```python
from build123d import *

# Parameters (mm, degrees)
F1_DEPTH       = 15
F1_DEPTH_BACK  = 5
F2_START       = 11
F2_DEPTH       = 4
F3_DEPTH       = 5
F4_D           = 3.8
F4_CSINK_D     = 8.5
F4_CSINK_ANGLE = 90
F5_SIZE        = 1.5


with BuildPart() as f1:
    # F0 (on Top) → F1 (new body, two sides)
    with BuildSketch(Plane.XY) as f1_sk:
        with BuildLine():
            ThreePointArc((7.3, 0), (0, -7.3), (-7.3, 0))
            Line((-7.3, 0), (-7.3, 8))
            Line((-7.3, 8), (-10.3, 8))
            Line((-10.3, 8), (-10.3, 0))
            ThreePointArc((-10.3, 0), (0, -10.3), (10.3, 0))
            Line((10.3, 0), (10.3, 8))
            Line((10.3, 8), (7.3, 8))
            Line((7.3, 8), (7.3, 0))
        make_face()
    extrude(amount=F1_DEPTH)
    extrude(f1_sk.sketch, amount=-F1_DEPTH_BACK)

    # F0 (on Top) → F2 (join)
    with BuildSketch(Plane.XY.offset(F2_START)):
        Polygon((-7.3, 8), (-7.3, 0), (-7, 0.7787641953), (-7, 8), align=None)
        Polygon((7, 0.7787641953), (7.3, 0), (7.3, 8), (7, 8), align=None)
    extrude(amount=F2_DEPTH)

    # F0 (on Top) → F3 (join)
    with BuildSketch(Plane.XY):
        Polygon((-7.3, 8), (-7.3, 0), (-7, 0.7787641953), (-7, 8), align=None)
        with BuildLine():
            Line((-7, 0.7787641953), (-7.3, 0))
            ThreePointArc((-7.3, 0), (0, -7.3), (7.3, 0))
            Line((7.3, 0), (7, 0.7787641953))
            Line((7, 0.7787641953), (7, 8))
            Line((7, 8), (7.3, 8))
            Line((7.3, 8), (10.3, 8))
            Line((10.3, 8), (10.3, 16))
            ThreePointArc((10.3, 16), (0, 26.3), (-10.3, 16))
            Line((-10.3, 16), (-10.3, 8))
            Line((-10.3, 8), (-7.3, 8))
            Line((-7.3, 8), (-7, 8))
            Line((-7, 8), (-7, 0.7787641953))
        make_face()
        Polygon((7, 0.7787641953), (7.3, 0), (7.3, 8), (7, 8), align=None)
    extrude(amount=-F3_DEPTH)

    # F4 (through all)
    with Locations(Plane.XY):
        with Locations((0, 16), (0, 0)):
            CounterSinkHole(F4_D / 2, F4_CSINK_D / 2, counter_sink_angle=F4_CSINK_ANGLE)

    # F5
    f5_edges = [f1.edges().sort_by_distance(p)[0] for p in [
        (-7, 8, 13),
        (7, 8, 13),
    ]]
    chamfer(f5_edges, length=F5_SIZE)


solid = f1.part
```
Check sheet for the modelled part. Datum: model origin and axes. Units: mm. A direction names the side the tool comes from. Coordinates: 2 decimals unless noted, no trailing zeros. Order: outer loops, then holes, each group sorted by start corner. A loop starts at its lowest first (then second) coordinate and runs counter-clockwise, first axis right, second up. Notation, with made-up numbers: (-36, 71.5) -> (-24, 71.5) arc R28 cw to (-24, 105.5) -> close; hole circle Ø10 at (-5, 14). An arc over 180 degrees is marked (long way). Write item = value, one per line. Start each with the question number.
1) Access from +Z, -Z, +X, -X, +Y, -Y to the whole of each face (thin tool, end or side, straight path). Record for faces 1 (the flat face through (0, 8, -5)), 2 (the cylindrical face through (1.9, 0.08, -3.69)), 3 (the flat face through (7.3, 3, 6)), 4 (the flat face through (-9, 8, 7)), 5 (the flat face through (-7.9, 7.4, 7.4)).
2) Go/stop test with flat-tipped pins: P1, Ø1, axis at x = 6.5, z = 5.5, coming from the -Y side; P2, Ø12, axis at y = 15.5, z = 11.5, coming from the -X side; P3, Ø4.5, axis at x = 0, y = 16, coming from the +Z side; P4, Ø0.9, axis at x = 9, z = 4, coming from the +Y side. Record where each tip stops, or that it passes through.
3) Cross-section at D-D (z = 13.75). Enter the section's corners in (x, y), then the cut area to 3 significant figures.
4) Cross-section at B-B (z = 5.25). Enter the section's corners in (x, y), then the cut area to 3 significant figures.
5) Material ranges on L1, parallel to Y at x = 0, z = -4.2; L2, parallel to X at y = 0, z = -3.5; L3, parallel to X at y = 5, z = 14, recorded low to high.
6) Cross-section at C-C (y = 9.5). Enter the section's corners in (x, z).
7) Mould release check, pull along Y, two halves, no side actions. Record for faces 6 (the flat face through (7.9, 7.4, 7.4)), 7 (the flat face through (-10.3, 5, 3)), 8 (the cylindrical face through (-0.2, -10.3, 5.1)), 9 (the conical face through (-0.929, 14.213, -2.236)): +Y half, -Y half, draft (parallel to the pull), parting line (faces both ways), or undercut.
8) Cross-section at A-A (x = 0). Enter the section's corners in (y, z).
Ans:
q1.face_1 = -Z, +X, -X, +Y, -Y
q1.face_2 = +Z, -Z
q1.face_3 = +Y
q1.face_4 = +Z, +X, -X, +Y
q1.face_5 = +Z, +Y
q2.P1 = -8.37
q2.P2 = through
q2.P3 = -2
q2.P4 = 8
q3.outline = (-10.3, 0) arc R10.3 ccw to (10.3, 0) -> (10.3, 8) -> (8.5, 8) -> (7, 6.5) -> (7, 0.78) -> (7.3, 0) arc R7.3 cw to (-7.3, 0) -> (-7, 0.78) -> (-7, 6.5) -> (-8.5, 8) -> (-10.3, 8) -> close
q3.area = 133 mm²
q4.outline = (-10.3, 0) arc R10.3 ccw to (10.3, 0) -> (10.3, 8) -> (8.5, 8) -> (7.3, 6.8) -> (7.3, 0) arc R7.3 cw to (-7.3, 0) -> (-7.3, 6.8) -> (-8.5, 8) -> (-10.3, 8) -> close
q4.area = 129 mm²
q5.L1 = -10.3 to -1.9, 1.9 to 14.1, 17.9 to 26.3
q5.L2 = -10.3 to -1.9, 1.9 to 10.3
q5.L3 = -10.3 to -7, 7 to 10.3
q6.outline = (-10.3, -5) -> (10.3, -5) -> (10.3, 0) -> (-10.3, 0) -> close
q7.face_6 = +Y half
q7.face_7 = draft
q7.face_8 = -Y half
q7.face_9 = undercut
q8.outline = (-10.3, -5) -> (-1.9, -5) -> (-1.9, -2.35) -> (-4.25, 0) -> (-7.3, 0) -> (-7.3, 15) -> (-10.3, 15) -> close; (1.9, -5) -> (14.1, -5) -> (14.1, -2.35) -> (11.75, 0) -> (4.25, 0) -> (1.9, -2.35) -> close; (17.9, -5) -> (26.3, -5) -> (26.3, 0) -> (20.25, 0) -> (17.9, -2.35) -> close
